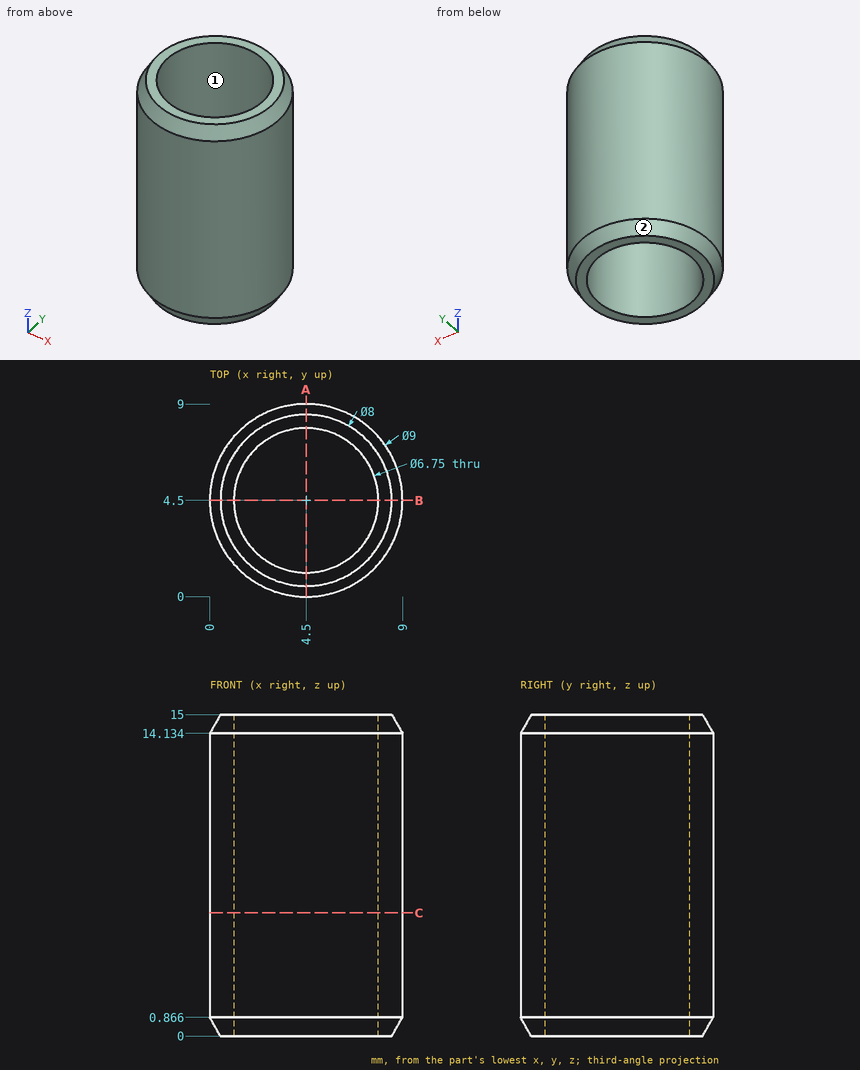
Verification items for this drawing (mm, ordinates from the low corner). Coordinates: 2 decimals unless noted, no trailing zeros. Write each loop counter-clockwise with the first axis right and the second up, starting at its lowest first coordinate (ties: lowest second). Pieces come first, ordered by that corner, then holes. Notation, with made-up numbers: M 52.25,25.5 L 101.25,25.5 A30 ccw 101.25,63.5 Z; hole C 26.25,37 d11. An arc over 180 degrees is marked long. Use CSV: the item, a comma, the result in double quotes.
Q1. Mould release check, pull along X, two halves, no side actions. Record for the marked faces 1 and 2: pulls with the +X half, pulls with the -X half, needs draft (parallel to the pull), parting line crosses it, or undercut.
Computed values:
face 1,"undercut"
face 2,"parting line crosses it"
Q2. Go/stop test with flat-tipped pins: P1, Ø1, axis at y = 5.5, z = 9, coming from the -X side; P2, Ø1.5, axis at x = 8, y = 8, coming from the -Z side. Record where each tip stops, or that it passes through.
Computed values:
P1,"x = 0.03"
P2,"z = 0.35"
Q3. Thickness scan on line 1 along Y through (x, z) = (4.5, 10.5) (3 decimals); line 2 along Y through (x, z) = (4, 8.5); line 3 along X through (y, z) = (5.75, 14.75) (3 decimals). Record the ranges inside material, lowest first. Write a range as [from, to].
Computed values:
line 1,"[0, 1.125], [7.875, 9]"
line 2,"[0.03, 1.16], [7.84, 8.97]"
line 3,"[0.549, 1.365], [7.635, 8.451]"
Q4. Section check C-C, the plane z = 5.75. Enter the section's corners in (x, y) (3 decimals), and give its area (3 significant figures).
Computed values:
outline,"C 4.5,4.5 d9; hole C 4.5,4.5 d6.75"
area,"27.8 mm²"
Q5. Section check A-A, the plane x = 4.5. Enter the section's corners in (y, z) (3 decimals).
Computed values:
outline,"M 0,0.866 L 0.5,0 L 1.125,0 L 1.125,15 L 0.5,15 L 0,14.134 Z; M 7.875,0 L 8.5,0 L 9,0.866 L 9,14.134 L 8.5,15 L 7.875,15 Z"
